The listing builds one solid part. Answer for the finished solid, in the listing's coordinates (mm). Give positions to 0.01 mm unless a question says otherwise; leave off trailing zeros. Write each loop counter-clockwise with the first axis right and the second up, starting at its lowest first coordinate (ties: lowest second). Pieces come first, ordered by that corner, then holes.
```python
from build123d import *

# Parameters (mm, degrees)
F0_W         = 25.4
F0_H         = 25.4
F0_R         = 6.35
F1_DEPTH     = 6.35
F2_SIZE      = 5.08
F3_T4_DEPTH  = 51.5282991577
F3_T9_DEPTH  = 51.5282991577
F3_T14_DEPTH = 51.5282991577
F3_T19_DEPTH = 51.5282991577
F3_T24_DEPTH = 51.5282991577
F3_T29_DEPTH = 51.5282991577
F3_T34_DEPTH = 51.5282991577
F3_T39_DEPTH = 51.5282991577
F3_T47_DEPTH = 51.5282991577
F3_T51_DEPTH = 51.5282991577
F3_T58_DEPTH = 51.5282991577
F3_T62_DEPTH = 51.5282991577
F3_T69_DEPTH = 51.5282991577
F3_T73_DEPTH = 51.5282991577
F3_T80_DEPTH = 51.5282991577
F3_T84_DEPTH = 51.5282991577


# Not quite as in the source:
# - a fillet or chamfer that OpenCascade refuses, or shapes differently, is made with other operations: its cross-section is extruded or revolved along the edge and cut away or added


with BuildPart() as f1:
    # F0 (on Top) → F1 (new body)
    with BuildSketch(Plane.XY):
        Polygon((12.7, 47.3970452561), (0, 25.4), (25.4, 25.4), align=None)
        with Locations((12.7, 12.7)):
            Rectangle(F0_W, F0_H)
        with Locations((12.7, 12.7)):
            Circle(F0_R, mode=Mode.SUBTRACT)
        Polygon((25.4, 25.4), (25.4, 0), (47.3970452561, 12.7), align=None)
        Polygon((25.4, 0), (0, 0), (12.7, -21.9970452561), align=None)
        Polygon((-21.9970452561, 12.7), (0, 0), (0, 25.4), align=None)
    extrude(amount=F1_DEPTH)

    # F2
    f2_edges = [f1.edges().sort_by_distance(p)[0] for p in [
        (6.35, 36.398523, 6.35),
        (-10.998523, 19.05, 6.35),
        (-10.998523, 6.35, 6.35),
        (6.35, -10.998523, 6.35),
        (19.05, -10.998523, 6.35),
        (36.398523, 6.35, 6.35),
        (36.398523, 19.05, 6.35),
        (19.05, 36.398523, 6.35),
        (6.35, 12.7, 6.35),
    ]]
    chamfer(f2_edges, length=F2_SIZE)

    # F3: chamfer of 5.08 on 9 edges, made by hand


with BuildPart() as f3_tool2:
    # F3_s3 → F3_t4 (new body)
    with BuildSketch(Plane(origin=(41.3624080422, -23.8805974175, 0), x_dir=(0, 0, 1), z_dir=(-0.8660254038, 0.5, 0))):
        Polygon((0, 29.6170452561), (5.08, 34.6970452561), (0, 34.6970452561), align=None)
    extrude(amount=F3_T4_DEPTH)

    split(bisect_by=Plane(origin=(30.0485226281, 17.3485226281, 0), x_dir=(0, 0, 1), z_dir=(0.8660254038, 0.5, 0)), keep=Keep.TOP)


with BuildPart() as f1_1:
    add(f1.part)

    # F3_t1: cut F3_tool2
    add(f3_tool2.part, mode=Mode.SUBTRACT)


with BuildPart() as f3_tool7:
    # F3_s8 → F3_t9 (new body)
    with BuildSketch(Plane(origin=(30.2305974175, 52.3609306703, 0), x_dir=(0, 0, 1), z_dir=(-0.5, -0.8660254038, 0))):
        Polygon((5.08, 12.7), (0, 7.62), (0, 12.7), align=None)
    extrude(amount=F3_T9_DEPTH)

    split(bisect_by=Plane(origin=(-10.9985226281, 19.05, 0), x_dir=(0, 0, 1), z_dir=(-0.5, 0.8660254038, 0)), keep=Keep.TOP)


with BuildPart() as f1_2:
    add(f1_1.part)

    # F3_t6: cut F3_tool7
    add(f3_tool7.part, mode=Mode.SUBTRACT)


with BuildPart() as f3_tool12:
    # F3_s13 → F3_t14 (new body)
    with BuildSketch(Plane(origin=(22.3124080422, 12.8820747894, 0), x_dir=(0, 0, 1), z_dir=(-0.8660254038, -0.5, 0))):
        Polygon((0, 16.9170452561), (5.08, 21.9970452561), (0, 21.9970452561), align=None)
    extrude(amount=F3_T14_DEPTH)

    split(bisect_by=Plane(origin=(-10.9985226281, 6.35, 0), x_dir=(0, 0, 1), z_dir=(-0.8660254038, 0.5, 0)), keep=Keep.TOP)


with BuildPart() as f1_3:
    add(f1_2.part)

    # F3_t11: cut F3_tool12
    add(f3_tool12.part, mode=Mode.SUBTRACT)


with BuildPart() as f3_tool17:
    # F3_s18 → F3_t19 (new body)
    with BuildSketch(Plane(origin=(-33.3109306703, 19.2320747894, 0), x_dir=(0, 0, 1), z_dir=(0.8660254038, -0.5, 0))):
        Polygon((0, -5.08), (5.08, 0), (0, 0), align=None)
    extrude(amount=F3_T19_DEPTH)

    split(bisect_by=Plane(origin=(0, 0, 0), x_dir=(0, 0, 1), z_dir=(-0.8660254038, -0.5, 0)), keep=Keep.TOP)


with BuildPart() as f1_4:
    add(f1_3.part)

    # F3_t16: cut F3_tool17
    add(f3_tool17.part, mode=Mode.SUBTRACT)


with BuildPart() as f3_tool22:
    # F3_s23 → F3_t24 (new body)
    with BuildSketch(Plane(origin=(-6.5320747894, 11.3138854141, 0), x_dir=(0, 0, 1), z_dir=(0.5, -0.8660254038, 0))):
        Polygon((0, -5.08), (5.08, 0), (0, 0), align=None)
    extrude(amount=F3_T24_DEPTH)

    split(bisect_by=Plane(origin=(0, 0, 0), x_dir=(0, 0, 1), z_dir=(-0.5, -0.8660254038, 0)), keep=Keep.TOP)


with BuildPart() as f1_5:
    add(f1_4.part)

    # F3_t21: cut F3_tool22
    add(f3_tool22.part, mode=Mode.SUBTRACT)


with BuildPart() as f3_tool27:
    # F3_s28 → F3_t29 (new body)
    with BuildSketch(Plane(origin=(-12.8820747894, -22.3124080422, 0), x_dir=(0, 0, 1), z_dir=(0.5, 0.8660254038, 0))):
        Polygon((0, 16.9170452561), (5.08, 21.9970452561), (0, 21.9970452561), align=None)
    extrude(amount=F3_T29_DEPTH)

    split(bisect_by=Plane(origin=(6.35, -10.9985226281, 0), x_dir=(0, 0, 1), z_dir=(0.5, -0.8660254038, 0)), keep=Keep.TOP)


with BuildPart() as f1_6:
    add(f1_5.part)

    # F3_t26: cut F3_tool27
    add(f3_tool27.part, mode=Mode.SUBTRACT)


with BuildPart() as f3_tool32:
    # F3_s33 → F3_t34 (new body)
    with BuildSketch(Plane(origin=(7.7361145859, 4.4664478386, 0), x_dir=(0, 0, 1), z_dir=(0.8660254038, 0.5, 0))):
        Polygon((0, 7.62), (5.08, 12.7), (0, 12.7), align=None)
    extrude(amount=F3_T34_DEPTH)

    split(bisect_by=Plane(origin=(19.05, -10.9985226281, 0), x_dir=(0, 0, 1), z_dir=(0.8660254038, -0.5, 0)), keep=Keep.TOP)


with BuildPart() as f1_7:
    add(f1_6.part)

    # F3_t31: cut F3_tool32
    add(f3_tool32.part, mode=Mode.SUBTRACT)


with BuildPart() as f3_tool37:
    # F3_s38 → F3_t39 (new body)
    with BuildSketch(Plane(origin=(1.8835521614, -3.2624080422, 0), x_dir=(0, 0, 1), z_dir=(-0.5, 0.8660254038, 0))):
        Polygon((5.08, 34.6970452561), (0, 29.6170452561), (0, 34.6970452561), align=None)
    extrude(amount=F3_T39_DEPTH)

    split(bisect_by=Plane(origin=(17.3485226281, 30.0485226281, 0), x_dir=(0, 0, 1), z_dir=(0.5, 0.8660254038, 0)), keep=Keep.TOP)


with BuildPart() as f1_8:
    add(f1_7.part)

    # F3_t36: cut F3_tool37
    add(f3_tool37.part, mode=Mode.SUBTRACT)

    # F3_s41 → F3_t42 (revolve, cut)
    with BuildSketch(Plane.XZ.offset(-12.7)):
        Polygon((24.13, 0), (19.05, 5.08), (19.05, 0), align=None)
    revolve(axis=Axis((12.7, 12.7, 0), (0, 0, 1)), mode=Mode.SUBTRACT)


with BuildPart() as f3_tool45:
    # F3_s46 → F3_t47 (new body)
    with BuildSketch(Plane(origin=(1.8835521614, -3.2624080422, 0), x_dir=(0, 0, 1), z_dir=(-0.5, 0.8660254038, 0))):
        Polygon((5.08, 34.6970452561), (0, 29.6170452561), (0, 34.6970452561), align=None)
    extrude(amount=F3_T47_DEPTH)

    split(bisect_by=Plane(origin=(17.3485226281, 30.0485226281, 0), x_dir=(0, 0, 1), z_dir=(-0.5, -0.8660254038, 0)), keep=Keep.TOP)


with BuildPart() as f3_tool49:
    # F3_s50 → F3_t51 (new body)
    with BuildSketch(Plane(origin=(41.3624080422, -23.8805974175, 0), x_dir=(0, 0, 1), z_dir=(-0.8660254038, 0.5, 0))):
        Polygon((0, 29.6170452561), (5.08, 34.6970452561), (0, 34.6970452561), align=None)
    extrude(amount=F3_T51_DEPTH)

    split(bisect_by=Plane(origin=(30.0485226281, 17.3485226281, 0), x_dir=(0, 0, 1), z_dir=(-0.8660254038, -0.5, 0)), keep=Keep.TOP)


with BuildPart() as f3_tool45_1:
    add(f3_tool45.part)

    # F3_t53: intersect F3_tool49
    add(f3_tool49.part, mode=Mode.INTERSECT)


with BuildPart() as f1_9:
    add(f1_8.part)

    # F3_t43: cut F3_tool45
    add(f3_tool45_1.part, mode=Mode.SUBTRACT)


with BuildPart() as f3_tool56:
    # F3_s57 → F3_t58 (new body)
    with BuildSketch(Plane(origin=(30.2305974175, 52.3609306703, 0), x_dir=(0, 0, 1), z_dir=(-0.5, -0.8660254038, 0))):
        Polygon((5.08, 12.7), (0, 7.62), (0, 12.7), align=None)
    extrude(amount=F3_T58_DEPTH)

    split(bisect_by=Plane(origin=(-10.9985226281, 19.05, 0), x_dir=(0, 0, 1), z_dir=(0.5, -0.8660254038, 0)), keep=Keep.TOP)


with BuildPart() as f3_tool60:
    # F3_s61 → F3_t62 (new body)
    with BuildSketch(Plane(origin=(22.3124080422, 12.8820747894, 0), x_dir=(0, 0, 1), z_dir=(-0.8660254038, -0.5, 0))):
        Polygon((0, 16.9170452561), (5.08, 21.9970452561), (0, 21.9970452561), align=None)
    extrude(amount=F3_T62_DEPTH)

    split(bisect_by=Plane(origin=(-10.9985226281, 6.35, 0), x_dir=(0, 0, 1), z_dir=(0.8660254038, -0.5, 0)), keep=Keep.TOP)


with BuildPart() as f3_tool56_1:
    add(f3_tool56.part)

    # F3_t64: intersect F3_tool60
    add(f3_tool60.part, mode=Mode.INTERSECT)


with BuildPart() as f1_10:
    add(f1_9.part)

    # F3_t54: cut F3_tool56
    add(f3_tool56_1.part, mode=Mode.SUBTRACT)


with BuildPart() as f3_tool67:
    # F3_s68 → F3_t69 (new body)
    with BuildSketch(Plane(origin=(-33.3109306703, 19.2320747894, 0), x_dir=(0, 0, 1), z_dir=(0.8660254038, -0.5, 0))):
        Polygon((0, -5.08), (5.08, 0), (0, 0), align=None)
    extrude(amount=F3_T69_DEPTH)

    split(bisect_by=Plane(origin=(0, 0, 0), x_dir=(0, 0, 1), z_dir=(0.8660254038, 0.5, 0)), keep=Keep.TOP)


with BuildPart() as f3_tool71:
    # F3_s72 → F3_t73 (new body)
    with BuildSketch(Plane(origin=(-6.5320747894, 11.3138854141, 0), x_dir=(0, 0, 1), z_dir=(0.5, -0.8660254038, 0))):
        Polygon((0, -5.08), (5.08, 0), (0, 0), align=None)
    extrude(amount=F3_T73_DEPTH)

    split(bisect_by=Plane(origin=(0, 0, 0), x_dir=(0, 0, 1), z_dir=(0.5, 0.8660254038, 0)), keep=Keep.TOP)


with BuildPart() as f3_tool67_1:
    add(f3_tool67.part)

    # F3_t75: intersect F3_tool71
    add(f3_tool71.part, mode=Mode.INTERSECT)


with BuildPart() as f1_11:
    add(f1_10.part)

    # F3_t65: cut F3_tool67
    add(f3_tool67_1.part, mode=Mode.SUBTRACT)


with BuildPart() as f3_tool78:
    # F3_s79 → F3_t80 (new body)
    with BuildSketch(Plane(origin=(-12.8820747894, -22.3124080422, 0), x_dir=(0, 0, 1), z_dir=(0.5, 0.8660254038, 0))):
        Polygon((0, 16.9170452561), (5.08, 21.9970452561), (0, 21.9970452561), align=None)
    extrude(amount=F3_T80_DEPTH)

    split(bisect_by=Plane(origin=(6.35, -10.9985226281, 0), x_dir=(0, 0, 1), z_dir=(-0.5, 0.8660254038, 0)), keep=Keep.TOP)


with BuildPart() as f3_tool82:
    # F3_s83 → F3_t84 (new body)
    with BuildSketch(Plane(origin=(7.7361145859, 4.4664478386, 0), x_dir=(0, 0, 1), z_dir=(0.8660254038, 0.5, 0))):
        Polygon((0, 7.62), (5.08, 12.7), (0, 12.7), align=None)
    extrude(amount=F3_T84_DEPTH)

    split(bisect_by=Plane(origin=(19.05, -10.9985226281, 0), x_dir=(0, 0, 1), z_dir=(-0.8660254038, 0.5, 0)), keep=Keep.TOP)


with BuildPart() as f3_tool78_1:
    add(f3_tool78.part)

    # F3_t86: intersect F3_tool82
    add(f3_tool82.part, mode=Mode.INTERSECT)


with BuildPart() as f1_12:
    add(f1_11.part)

    # F3_t76: cut F3_tool78
    add(f3_tool78_1.part, mode=Mode.SUBTRACT)


solid = f1_12.part
```
Item 1: Each of these flat-tipped pins is pushed along its axis until it touches: P1, Ø2, axis at x = 36, z = 5, coming from the +Y side; P2, Ø2, axis at y = -8, z = 5.5, coming from the +X side; P3, Ø10, axis at x = 30.5, y = 2, coming from the +Z side. Where does it stop, or does it pass through?
Conclusion:
P1: stops at y = 16.26
P2: stops at x = 17.19
P3: stops at z = 5.45
Item 2: Determine the mould class of faces 1 (the face through (6.97, 30.53, 1.61)), 2 (the face through (32.481, 8.147, 1.565)), 3 (the face through (6.03, 7.58, 3.02)) for opening direction X: pulls with the +X half, pulls with the -X half, needs draft (parallel to the pull), parting line crosses it, or undercut.
Conclusion:
face 1: pulls with the -X half
face 2: pulls with the +X half
face 3: undercut
Item 3: A cutting plane is placed at D-D, the plane x = 38. Give the vertices of the cut face in (y, z) (3 decimals), plus the area to 3 significant figures.
Conclusion:
outline: (9.474, 3.175) - (12.7, 0.381) - (15.926, 3.175) - (12.7, 5.969) - close
area: 18.0 mm2
Item 4: A cutting plane is placed at B-B, the plane x = 25. Give the vertices of the cut face in (y, z) (3 decimals).
Conclusion:
outline: (1.969, 3.175) - (5.635, 0) - (19.765, 0) - (23.431, 3.175) - (19.765, 6.35) - (5.635, 6.35) - close
Item 5: A cutting plane is placed at C-C, the plane y = 31.5. Give the vertices of the cut face in (x, z) (3 decimals), plus the area to 3 significant figures.
Conclusion:
outline: (5.722, 3.175) - (9.388, 0) - (16.012, 0) - (19.678, 3.175) - (16.012, 6.35) - (9.388, 6.35) - close
area: 65.3 mm2
Item 6: Consider probe 1 along Y at (x, z) = (10, 4.75); probe 2 along X at (y, z) = (19.5, 4); probe 3 along X at (y, z) = (15, 1.25). Determine where each line is inside the solid, lowest interval first.
Conclusion:
probe 1: y = -10.36 to 3.25, 22.15 to 35.76
probe 2: x = -4.76 to 6.68, 18.72 to 30.16
probe 3: x = -10.35 to 2.78, 22.62 to 35.75
Item 7: A cutting plane is placed at A-A, the plane z = 1.25. Give the vertices of the cut face in (x, y), plus the area to 3 significant figures.
Conclusion:
outline: (-14.34, 12.7) - (2.8, 2.8) - (12.7, -14.34) - (22.6, 2.8) - (39.74, 12.7) - (22.6, 22.6) - (12.7, 39.74) - (2.8, 22.6) - close; hole circle Ø20.36 at (12.7, 12.7)
area: 745 mm2
